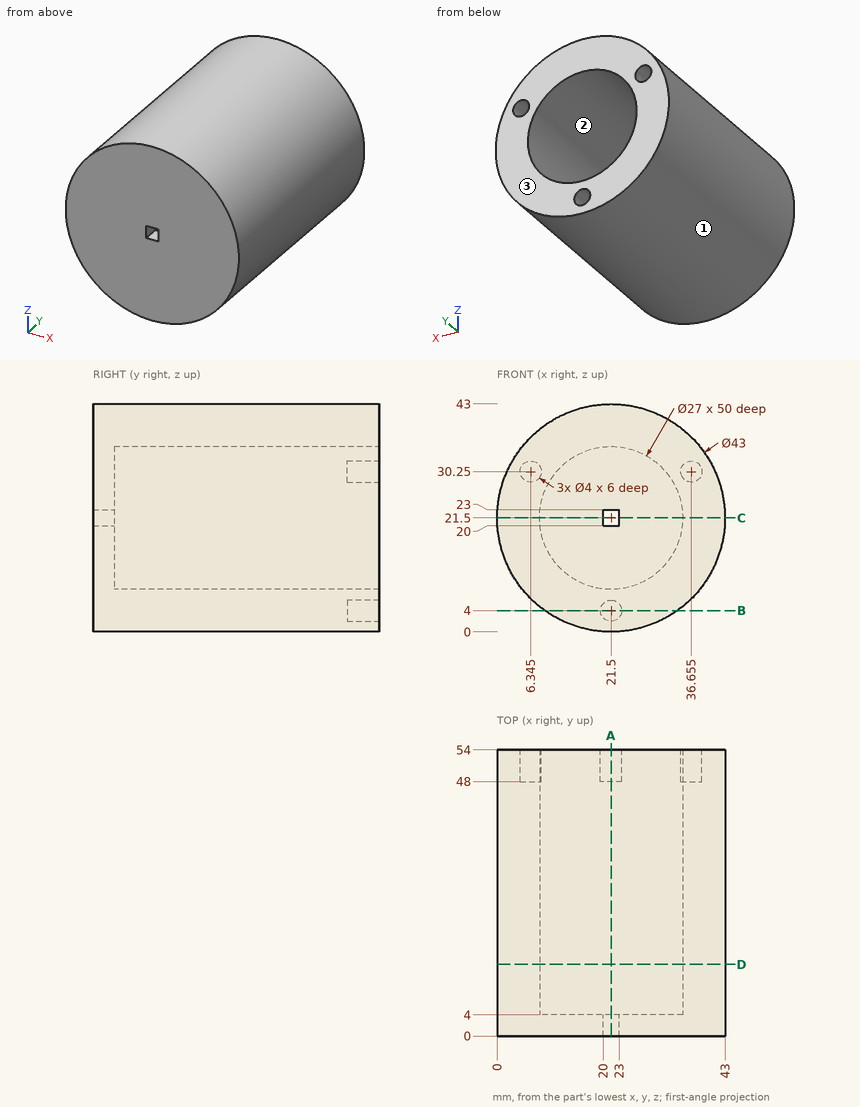
Part print with two shaded views. Sizes in mm from the minimum x, y, z corner. Coordinates: 2 decimals unless noted, no trailing zeros. Order: outer loops, then holes, each group sorted by start corner. A loop starts at its lowest first (then second) coordinate and runs counter-clockwise, first axis right, second up. Notation, with made-up numbers: (25, 55.25) - (71, 55.25) arc R31 ccw to (71, 83.25) - close; hole circle Ø7 at (-31.75, 66.5). An arc over 180 degrees is marked (long way). Write item = value, one per line. Start each with the question number.
1) Two-plate mould, pull along X, no slides. Class the marked faces 1, 2 and 3: pulls with the +X half, pulls with the -X half, needs draft (parallel to the pull), parting line crosses it, or undercut.
2) Saw through at A-A on x = 21.5. Write the cut outline in (y, z).
3) Saw through at B-B on z = 4. Write the cut outline in (x, y).
4) Saw through at C-C on z = 21.5. Write the cut outline in (x, y), then the cut area to 3 significant figures.
5) Wall check: line 1 along X through (y, z) = (49, 30); line 2 along Y through (x, z) = (22, 17); line 3 along X through (y, z) = (41, 13.5) (1 decimal). Give the ranges that are in metal, low to high. Write a range as from..to.
6) Saw through at D-D on y = 13.5. Write the cut outline in (x, z).
7) Flat gauge pins, fed straight in: pin 1 Ø4 at (y, z) = (12.5, 36) entering from +X; pin 2 Ø2 at (x, y) = (9.5, 30) entering from +Z; pin 3 Ø4 at (x, y) = (38.5, 23.5) entering from -Z. Where does each tip first touch, or does it go through?
From the geometry:
q1.face_1 = parting line crosses it
q1.face_2 = undercut
q1.face_3 = needs draft
q2.outline = (0, 0) - (54, 0) - (54, 2) - (48, 2) - (48, 6) - (54, 6) - (54, 8) - (4, 8) - (4, 20) - (0, 20) - close; (0, 23) - (4, 23) - (4, 35) - (54, 35) - (54, 43) - (0, 43) - close
q3.outline = (9.01, 0) - (33.99, 0) - (33.99, 54) - (23.5, 54) - (23.5, 48) - (19.5, 48) - (19.5, 54) - (9.01, 54) - close
q4.outline = (0, 0) - (20, 0) - (20, 4) - (8, 4) - (8, 54) - (0, 54) - close; (23, 0) - (43, 0) - (43, 54) - (35, 54) - (35, 4) - (23, 4) - close
q4.area = 960 mm^2
q5.line_1 = 1.75..4.36, 8.33..11.01, 31.99..34.67, 38.64..41.25
q5.line_2 = 0..4
q5.line_3 = 1.5..10.6, 32.4..41.5
q6.outline = circle Ø43 at (21.5, 21.5); hole circle Ø27 at (21.5, 21.5)
q7.pin_1 = 38.99
q7.pin_2 = 39.97
q7.pin_3 = 6.1
